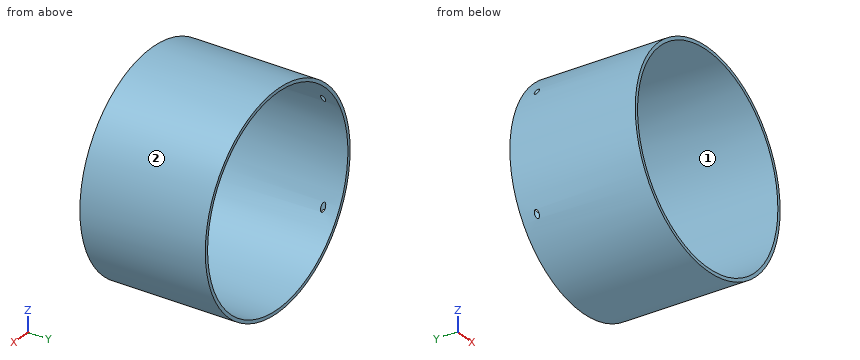
```python
from build123d import *

# Parameters (mm, degrees)
SKETCH1_R               = 101.6
SKETCH1_R_2             = 95.25
BOSS_EXTRUDE1_DEPTH     = 25.4
SKETCH2_R               = 3.175
CUT_EXTRUDE1_DEPTH      = 102.6
CUT_EXTRUDE1_DEPTH_BACK = 102.6
SKETCH5_R               = 101.6
SKETCH5_R_2             = 98.425
BOSS_EXTRUDE2_DEPTH     = 146.05
SKETCH9_R               = 2.1
CUT_EXTRUDE5_DEPTH      = 204.2000001
SKETCH10_R              = 101.6
CUT_EXTRUDE6_DEPTH      = 50.8


with BuildPart() as part:
    # Sketch1 → Boss-Extrude1 (new body)
    with BuildSketch(Plane(origin=(0, 0, 0), x_dir=(1, 0, 0), z_dir=(0, 1, 0))):
        Circle(SKETCH1_R)
        Circle(SKETCH1_R_2, mode=Mode.SUBTRACT)
    extrude(amount=BOSS_EXTRUDE1_DEPTH)

    # Sketch2 → Cut-Extrude1 (cut, two sides)
    with BuildSketch(Plane.XY) as cut_extrude1_sk:
        with Locations((0, 12.7)):
            Circle(SKETCH2_R)
    extrude(amount=CUT_EXTRUDE1_DEPTH, mode=Mode.SUBTRACT)
    extrude(cut_extrude1_sk.sketch, amount=-CUT_EXTRUDE1_DEPTH_BACK, mode=Mode.SUBTRACT)

    # Sketch5 → Boss-Extrude2 (add)
    with BuildSketch(Plane(origin=(0, 25.4, 0), x_dir=(1, 0, 0), z_dir=(0, 1, 0))):
        Circle(SKETCH5_R)
        Circle(SKETCH5_R_2, mode=Mode.SUBTRACT)
    extrude(amount=BOSS_EXTRUDE2_DEPTH)

    # Sketch9 → Cut-Extrude5 (cut, through all)
    with BuildSketch(Plane.XY.offset(101.6)):
        with Locations((-85.075, 156.8)):
            Circle(SKETCH9_R)
    extrude(amount=-CUT_EXTRUDE5_DEPTH, mode=Mode.SUBTRACT)

    # Sketch10 → Cut-Extrude6 (cut)
    with BuildSketch(Plane(origin=(0, 0, 0), x_dir=(-1, 0, 0), z_dir=(0, -1, 0))):
        Circle(SKETCH10_R)
    extrude(amount=-CUT_EXTRUDE6_DEPTH, mode=Mode.SUBTRACT)


solid = part.part
```
Geometry: final body of the model. Coordinates: model frame, mm. Face numbers are marked on the shaded views. Round coordinates to 2 decimals unless told otherwise and drop trailing zeros. Order: outer loops, then holes, each group sorted by start corner. A loop starts at its lowest first (then second) coordinate and runs counter-clockwise, first axis right, second up. Notation, with made-up numbers: (62.25, 22.25) -> (81.25, 22.25) arc R20 ccw to (81.25, 42.25) -> close; hole circle Ø1 at (-13, -1.75). An arc over 180 degrees is marked (long way). Use one line per item in the form item = value. Start each with the question number.
1. Cut plane C-C (y = 62.5). Return the cut outline in (x, z) (3 decimals).
2. Cut plane A-A (x = 0). Return the cut outline in (y, z) (3 decimals), then the cut area to 3 significant figures.
3. Pin query (flat end, axial travel): pin 1 Ø2 at (y, z) = (89, -20.5) entering from -X; pin 2 Ø3.5 at (x, y) = (-85.075, 156.8) entering from -Z; pin 3 Ø1 at (x, y) = (28, 93.5) entering from -Z; pin 4 Ø2 at (y, z) = (92.5, 61) entering from -X. Return the tip coordinate at first contact, or that it passes through.
4. Cut plane B-B (z = 0). Return the cut outline in (x, y) (3 decimals), then the cut area to 3 significant figures.
5. Line query: probe 1 along Z at (x, y) = (-2, 85); probe 2 along X at (y, z) = (70.5, 2.5); probe 3 along X at (y, z) = (84.5, 69.5). Output: solid intervals per line, ascending.
6. Draft query along Z for the marked faces 1 and 2. Return one class per face: pulls with the +Z half, pulls with the -Z half, needs draft (parallel to the pull), parting line crosses it, or undercut.
Solution:
q1.outline = circle Ø203.2 at (0, 0); hole circle Ø196.85 at (0, 0)
q2.outline = (50.8, -101.6) -> (171.45, -101.6) -> (171.45, -98.425) -> (50.8, -98.425) -> close; (50.8, 98.425) -> (171.45, 98.425) -> (171.45, 101.6) -> (50.8, 101.6) -> close
q2.area = 766 mm^2
q3.pin_1 = -99.71
q3.pin_2 = through
q3.pin_3 = -97.81
q3.pin_4 = -81.99
q4.outline = (-101.6, 50.8) -> (-98.425, 50.8) -> (-98.425, 171.45) -> (-101.6, 171.45) -> close; (98.425, 50.8) -> (101.6, 50.8) -> (101.6, 171.45) -> (98.425, 171.45) -> close
q4.area = 766 mm^2
q5.probe_1 = -101.58 to -98.4, 98.4 to 101.58
q5.probe_2 = -101.57 to -98.39, 98.39 to 101.57
q5.probe_3 = -74.11 to -69.69, 69.69 to 74.11
q6.face_1 = undercut
q6.face_2 = parting line crosses it
